Autodesk Inventor part; units mm, degrees
ref_plane "YZ Plane" through (0, 0, 0) normal (1, 0, 0) x (0, 1, 0)
ref_plane "XZ Plane" through (0, 0, 0) normal (0, 1, 0) x (-1, 0, 0)
ref_plane "XY Plane" through (0, 0, 0) normal (0, 0, 1) x (1, 0, 0)
sketch "Sketch1" plane through (0, 0, 0) normal (0, 1, 0) x (-1, 0, 0)
  circle A0 centre (0, 0) radius 59
  circle A1 centre (0, 0) radius 81
  circle A2 centre (0, 0) radius 87.5
  circle A3 centre (0, 81) radius 2.25
  circle A4 centre (0, -81) radius 2.25
  line L0 (90, -56) -> (15, -56)
  line L1 (10, -51) -> (10, 51)
  line L2 (15, 56) -> (90, 56)
  line L3 (90, 56) -> (90, -56)
  line L4 (90, -56) -> (10, 56) construction
  line L5 (10, -56) -> (90, 56) construction
  arc A5 (10, -51) -> (15, -56) centre (15, -51) ccw
  arc A6 (15, 56) -> (10, 51) centre (15, 51) ccw
  line L6 (0, 103.0841) -> (0, -103.0841)
  line L7 (-90, -56) -> (-15, -56)
  line L8 (-10, -51) -> (-10, 51)
  line L9 (-15, 56) -> (-90, 56)
  line L10 (-90, 56) -> (-90, -56)
  arc A7 (-15, -56) -> (-10, -51) centre (-15, -51) ccw
  arc A8 (-10, 51) -> (-15, 56) centre (-15, 51) ccw
  point P0 (50, 0)
  point P1 (90, 0)
  point P2 (10, 0)
  point P3 (56.2614, -45.3902)
  point P4 (56.2614, 63.4399)
  point P5 (76.2614, 44.4685)
  point P6 (76.2614, -26.4188)
  point P7 (63.4942, 65.0248)
  point P8 (63.4942, -46.9752)
  point P9 (18.5742, -56)
  point P10 (18.5742, 56)
  point P11 (67.2328, 56)
  point P12 (-67.2328, 56)
  point P13 (-58.5235, 56)
  point P14 (-58.5235, -56)
  point P15 (-67.2328, -56)
  point P16 (67.2328, -56)
  dimension "d0" = 118
  dimension "d1" = 162
  dimension "d2" = 175
  dimension "d3" = 4.5
  dimension "d4" = 4.5
  dimension "d5" = 112
  dimension "d6" = 80
  dimension "d7" = 10
  dimension "d8" = 5
  dimension "d9" = 0
  dimension "d10" = 0
  dimension "d11" = 56
extrude "Extrusion1" add sketch "Sketch1" along normal blind 5 contours A0 L6 A3 A1 L2 | L0 A1 A4 L6 A0 | A0 L9 A1 A3 L6 | A1 A3 L6 A2 L2 | L6 A4 A1 L7 A0 | L0 A2 L6 A4 A1 | A0 L7 A1 L9 | L9 A2 L6 A3 A1 | A1 A4 L6 A2 L7
chamfer "Chamfer1" distance 8 angle 45 2 edges at (67.2328, 2.5, 56) (67.2328, 2.5, -56)
fillet "Fillet1" radius 5 4 edges at (61.8372, 2.5, -61.9065) (59.2328, 2.5, 56) (61.8372, 2.5, 61.9065) (59.2328, 2.5, -56)
properties part number "Cylinder Segment Holder Both Cameras"
Verification items for the finished model (mm, model axes). A direction names the side the tool comes from. Give positions to 0.01 mm unless a question says otherwise; leave off trailing zeros. Write each loop counter-clockwise with the first axis right and the second up, starting at its lowest first coordinate (ties: lowest second). Pieces come first, ordered by that corner, then holes. Notation, with made-up numbers: (-40, 35.25) - (-12, 35.25) arc R14 ccw to (-12, 61.25) - close; hole circle Ø6 at (81.25, 29.25). An arc over 180 degrees is marked (long way). Answer as CSV lines item,"result". Start each with the question number.
1. Sectioned sample at A-A (x = 0). Record the boundary of the cut face in (y, z).
2. Set-up check for faces 5 (the face through (80.995, 2.465, -0.866)), 6 (the face through (-43, 2, 56)): record each of +Z, -Z, +X, -X, +Y, -Y from which the full face is reachable in a straight line by a thin tool's end or side.
3. Sectioned sample at B-B (y = 1.4). Record the boundary of the cut face in (x, z), then the cut area to 3 significant figures.
4. Thickness scan on line 1 (Z direction, x = 0, y = 3.2); line 2 (Z direction, x = 10.5, y = 1.6); line 3 (Z direction, x = -42, y = 3.3). Record the ranges inside material, lowest first.
5. Draft check along X on faces 1 (the face through (58.98, 2.46, -1.56)), 2 (the face through (-43, 2, -56)), 3 (the face through (-6.789, 2.465, -87.236)), 4 (the face through (60.735, 2.465, -61.786)). Enter one of: pulls with the +X half, pulls with the -X half, needs draft (parallel to the pull), parting line crosses it, or undercut.
6. Sectioned sample at D-D (x = -26.5). Record the boundary of the cut face in (y, z), then the cut area to 3 significant figures.
7. Sectioned sample at C-C (z = 81). Record the boundary of the cut face in (x, y).
8. Depth check by flat-ended pin: pin 1 (3.5 mm diameter, centred on x = 0, z = -81, fed in from +Y); pin 2 (2 mm diameter, centred on x = -18.5, y = 2, fed in from -Z); pin 3 (1 mm diameter, centred on x = 3, y = 3, fed in from +Z); pin 4 (1.5 mm diameter, centred on y = 4, z = -5.5, fed in from -X). Enter the tip coordinate at first touch or a pass-through.
Derived:
1,outline,"(0, -87.5) - (5, -87.5) - (5, -83.25) - (0, -83.25) - close; (0, -78.75) - (5, -78.75) - (5, -59) - (0, -59) - close; (0, 59) - (5, 59) - (5, 78.75) - (0, 78.75) - close; (0, 83.25) - (5, 83.25) - (5, 87.5) - (0, 87.5) - close"
2,face 5,"+X, +Y, -Y"
2,face 6,"-X, +Y, -Y"
3,outline,"(-67.23, -56) arc R87.5 ccw to (59.23, -64.4) arc R5 ccw to (60.42, -58.7) - (60.11, -57.99) arc R5 ccw to (58.52, -56) arc R81 ccw to (58.52, 56) arc R5 ccw to (60.11, 57.99) - (60.42, 58.7) arc R5 ccw to (59.23, 64.4) arc R87.5 ccw to (-67.23, 56) - (-18.57, 56) arc R59 cw (long way) to (-18.57, -56) - close; hole circle Ø4.5 at (0, -81); hole circle Ø4.5 at (0, 81)"
3,area,"8,550 mm²"
4,line 1,"-87.5 to -83.25, -78.75 to -59, 59 to 78.75, 83.25 to 87.5"
4,line 2,"-86.87 to -58.06, 58.06 to 86.87"
4,line 3,"-76.76 to -56, 56 to 76.76"
5,face 1,"undercut"
5,face 2,"needs draft"
5,face 3,"parting line crosses it"
5,face 4,"pulls with the +X half"
6,outline,"(0, -83.39) - (5, -83.39) - (5, -56) - (0, -56) - close; (0, 56) - (5, 56) - (5, 83.39) - (0, 83.39) - close"
6,area,"274 mm²"
7,outline,"(-33.09, 0) - (-2.25, 0) - (-2.25, 5) - (-33.09, 5) - close; (2.25, 0) - (33.09, 0) - (33.09, 5) - (2.25, 5) - close"
8,pin 1,"through"
8,pin 2,"z = -85.73"
8,pin 3,"z = 87.46"
8,pin 4,"x = 58.67"
